Geometry check sheet. Reference: the model listing, model coordinates, mm. Face numbers are marked on the shaded views. Coordinates: 2 decimals unless noted, no trailing zeros. Write each loop counter-clockwise with the first axis right and the second up, starting at its lowest first coordinate (ties: lowest second). Pieces come first, ordered by that corner, then holes. Notation, with made-up numbers: M -18.5,-29 L 21.5,-29 A21 ccw 21.5,-14 Z; hole C 62,44 d11. An arc over 180 degrees is marked long. Write item = value, one per line. Start each with the question number.
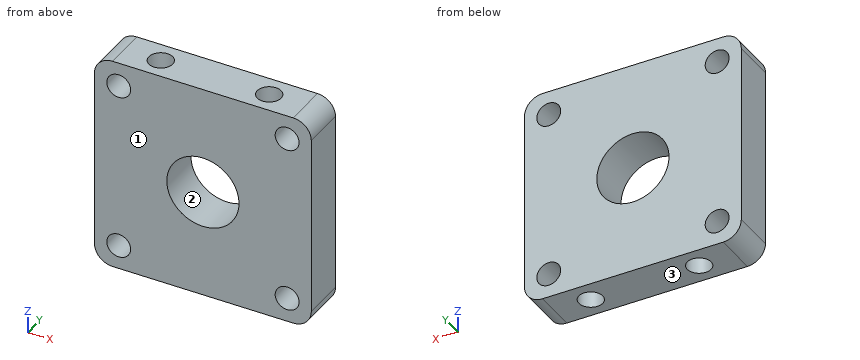
Autodesk Inventor part; units mm, degrees
ref_plane "YZ Plane" through (0, 0, 0) normal (1, 0, 0) x (0, 1, 0)
ref_plane "XZ Plane" through (0, 0, 0) normal (0, 1, 0) x (-1, 0, 0)
ref_plane "XY Plane" through (0, 0, 0) normal (0, 0, 1) x (1, 0, 0)
sketch "Sketch1" plane through (0, 0, 0) normal (0, 1, 0) x (-1, 0, 0)
  line L0 (16.6369, 20.0223) -> (-15.1131, 20.0223)
  line L1 (-18.2881, 16.8473) -> (-18.2881, -14.9027)
  line L2 (-15.1131, -18.0777) -> (16.6369, -18.0777)
  line L3 (19.8119, -14.9027) -> (19.8119, 16.8473)
  arc A0 (19.8119, 16.8473) -> (16.6369, 20.0223) centre (16.6369, 16.8473) ccw
  arc A1 (-18.2881, -14.9027) -> (-15.1131, -18.0777) centre (-15.1131, -14.9027) ccw
  arc A2 (16.6369, -18.0777) -> (19.8119, -14.9027) centre (16.6369, -14.9027) ccw
  arc A3 (-15.1131, 20.0223) -> (-18.2881, 16.8473) centre (-15.1131, 16.8473) ccw
  point P0 (0, 0)
  dimension "d0" = 38.1
  dimension "d1" = 3.175
extrude "Extrusion1" add sketch "Sketch1" along normal blind 7.62
sketch "Sketch2" plane through (0, 7.62, 0) normal (0, 1, 0) x (1, 0, 0)
  line L0 (-19.8119, 14.9027) -> (-19.8119, -16.8473)
  line L1 (-16.6369, -20.0223) -> (15.1131, -20.0223)
  line L2 (15.1131, 18.0777) -> (-16.6369, 18.0777)
  line L3 (18.2881, -16.8473) -> (18.2881, 14.9027)
  point P0 (0, 0)
  point P1 (-15.5619, -15.7723)
  point P2 (-15.5619, 13.8277)
  point P3 (14.0381, 13.8277)
  point P4 (14.0381, -15.7723)
  dimension "d4" = 4.25
  dimension "d5" = 4.25
  dimension "d6" = 4.25
  dimension "d7" = 4.25
  dimension "d8" = 4.25
  dimension "d9" = 4.25
  dimension "d10" = 4.25
  dimension "d11" = 4.25
hole "Hole1" at (-15.5619, 7.62, 15.7723) at (-15.5619, 7.62, -13.8277) at (14.0381, 7.62, -13.8277) at (14.0381, 7.62, 15.7723) direction (0, -1, 0) diameter 4.2 end through all
sketch "Sketch3" plane through (0, 7.62, 0) normal (0, 1, 0) x (1, 0, 0)
  line L0 (-19.8119, 14.9027) -> (-19.8119, -16.8473) construction
  line L1 (-19.8119, -0.9723) -> (18.2881, -0.9723) construction
  line L2 (18.2881, -16.8473) -> (18.2881, 14.9027) construction
  point P0 (0, 0)
  point P1 (-0.7619, -0.9723)
  point P2 (-0.7619, -0.9723)
hole "Hole2" at (-0.7619, 7.62, 0.9723) direction (0, -1, 0) diameter 12.7 end through all
sketch "Sketch4" plane through (-16.6369, 0, 20.0223) normal (0, 0, 1) x (1, 0, 0)
  line L0 (31.75, 0) -> (31.75, 7.62) construction
  line L1 (31.75, 3.81) -> (0, 3.81) construction
  line L2 (0, 0) -> (0, 7.62) construction
  line L3 (-3.175, 0) -> (-3.175, 7.62) construction
  line L4 (34.925, 0) -> (34.925, 7.62) construction
  point P0 (16.6369, 0)
  point P1 (6.35, 3.81)
  point P2 (25.4, 3.81)
  dimension "d26" = 9.525
  dimension "d27" = 9.525
hole "Hole3" at (-10.2869, 3.81, 20.0223) at (8.7631, 3.81, 20.0223) direction (0, 0, -1) diameter 4.2 depth 7.62 tip angle 118
sketch "Sketch5" plane through (15.1131, 0, -18.0777) normal (0, 0, -1) x (-1, 0, 0)
  line L0 (-3.175, 0) -> (-3.175, 7.62) construction
  line L1 (34.925, 0) -> (34.925, 7.62) construction
  line L2 (31.75, 0) -> (31.75, 7.62) construction
  line L3 (0, 0) -> (0, 7.62) construction
  line L4 (0, 0) -> (0, 7.62) construction
  line L5 (0, 3.81) -> (31.75, 3.81) construction
  line L6 (31.75, 0) -> (31.75, 7.62) construction
  point P0 (15.1131, 0)
  point P1 (6.35, 3.81)
  point P2 (25.4, 3.81)
  dimension "d35" = 9.525
  dimension "d36" = 9.525
hole "Hole4" at (8.7631, 3.81, -18.0777) at (-10.2869, 3.81, -18.0777) direction (0, 0, 1) diameter 4.2 depth 7.62 tip angle 118
properties part number "Bearing_Block" material "Steel, Mild"
Q1. Scan lines: L1, parallel to X at y = 3.81, z = -15.25; L2, parallel to Z at x = -1, y = 3; L3, parallel to X at y = 3.81, z = 18.25. Record each from-to range of solid material in increasing order.
Q2. Cross-section at A-A on x = -16. Enter the section's corners in (y, z).
Q3. Cross-section at B-B on z = 0. Enter the section's corners in (x, y).
Q4. Cross-section at C-C on x = 2.5. Enter the section's corners in (y, z).
Q5. Gauge pin test, flat ends, axial feed: pin 1 (1 mm diameter, centred on x = -12.5, z = -8, fed in from -Y); pin 2 (3.5 mm diameter, centred on x = 14.04, z = -13.83, fed in from -Y). Record the tip position at first contact, or that the pin passes through.
Q6. Draft check along Z on the marked faces 1, 2 and 3. Enter one of: pulls with the +Z half, pulls with the -Z half, needs draft (parallel to the pull), parting line crosses it, or undercut.
Q7. Cross-section at D-D on y = 7. Enter the section's corners in (x, z) (3 decimals), and give its area (3 significant figures).
Values found:
q1.L1 = -19.79 to -17.11, -14.02 to -12.39, -8.19 to 6.66, 10.86 to 12.49, 15.58 to 18.27
q1.L2 = -18.08 to -5.37, 7.32 to 20.02
q1.L3 = -19.49 to -12.39, -8.19 to 6.66, 10.86 to 17.96
q2.outline = M 0,-18.08 L 7.62,-18.08 L 7.62,-15.88 L 0,-15.88 Z; M 0,-11.77 L 7.62,-11.77 L 7.62,13.72 L 0,13.72 Z; M 0,17.83 L 7.62,17.83 L 7.62,20.02 L 0,20.02 Z
q3.outline = M -19.81,0 L -7.04,0 L -7.04,7.62 L -19.81,7.62 Z; M 5.51,0 L 18.29,0 L 18.29,7.62 L 5.51,7.62 Z
q4.outline = M 0,-18.08 L 7.62,-18.08 L 7.62,-4.48 L 0,-4.48 Z; M 0,6.42 L 7.62,6.42 L 7.62,20.02 L 0,20.02 Z
q5.pin_1 = 0
q5.pin_2 = through
q6.face_1 = needs draft
q6.face_2 = undercut
q6.face_3 = pulls with the -Z half
q7.outline = M -19.812,-14.903 A3.175 ccw -16.637,-18.078 L 15.113,-18.078 A3.175 ccw 18.288,-14.903 L 18.288,16.847 A3.175 ccw 15.113,20.022 L -16.637,20.022 A3.175 ccw -19.812,16.847 Z; hole C -15.562,-13.828 d4.2; hole C -15.562,15.772 d4.2; hole C -0.762,0.972 d12.7; hole C 14.038,-13.828 d4.2; hole C 14.038,15.772 d4.2
q7.area = 1,260 mm²
